Can you work these out from the model? Positions are in its coordinate system, mm. A direction names the side the tool comes from. Give positions to 0.01 mm unless a question says otherwise; leave off trailing zeros. Loops run counter-clockwise (first coordinate to the right, second up) from the corner with the lowest first, then second, coordinate; pieces in that order, holes last. Notation, with made-up numbers: (6.5, 57) -> (39.5, 57) arc R21 cw to (39.5, 94) -> close; hole circle Ø9 at (-36.75, 71.25). An arc over 180 degrees is marked (long way). Use CSV: the item, a comma, the result in double quotes.
from build123d import *

# Parameters (mm, degrees)
F1_DEPTH  = 35
F2_R      = 1
F4_DEPTH  = 25
F6_DEPTH  = 25
F8_DEPTH  = 25
F10_DEPTH = 25


with BuildPart() as f1:
    # F0 (on Top) → F1 (new body)
    with BuildSketch(Plane.XY):
        Polygon((1.5, 17.5), (1.5, 112.5), (-1.5, 112.5), (-1.5, 17.5), (-74, 17.5), (-74, 14.5), (-1.5, 14.5), (-1.5, -14.5), (-74, -14.5), (-74, -17.5), (-1.5, -17.5), (-1.5, -112.5), (1.5, -112.5), (1.5, -17.5), (74, -17.5), (74, -14.5), (1.5, -14.5), (1.5, 14.5), (74, 14.5), (74, 17.5), align=None)
    extrude(amount=F1_DEPTH)

    # F2
    f2_edges = [f1.edges().sort_by_distance(p)[0] for p in [
        (-37.75, 14.5, 35),
        (-1.5, 65, 35),
        (-37.75, 17.5, 35),
        (1.5, 65, 35),
        (37.75, 17.5, 35),
        (37.75, 14.5, 35),
        (1.5, 0, 35),
        (-1.5, 0, 35),
        (-37.75, -14.5, 35),
        (-37.75, -17.5, 35),
        (37.75, -14.5, 35),
        (37.75, -17.5, 35),
        (-1.5, -65, 35),
        (1.5, -65, 35),
    ]]
    fillet(f2_edges, radius=F2_R)

    # F3 (on face) → F4 (cut)
    with BuildSketch(Plane.XZ.offset(17.5)):
        with BuildLine():
            ThreePointArc((-46.6319660113, 34), (-37.75, 25.1180339887), (-28.8680339887, 34))
            Line((-28.8680339887, 34), (-46.6319660113, 34))
        make_face()
        with BuildLine():
            Line((-46.6319660113, 34), (-28.8680339887, 34))
            ThreePointArc((-28.8680339887, 34), (-37.75, 42.8819660113), (-46.6319660113, 34))
        make_face()
    extrude(amount=-F4_DEPTH, mode=Mode.SUBTRACT)

    # F5 (on face) → F6 (cut)
    with BuildSketch(Plane.XZ.offset(-14.5)):
        with BuildLine():
            ThreePointArc((-47.75, 34), (-37.75, 24), (-27.75, 34))
            Line((-27.75, 34), (-47.75, 34))
        make_face()
        with BuildLine():
            Line((-47.75, 34), (-27.75, 34))
            ThreePointArc((-27.75, 34), (-37.75, 44), (-47.75, 34))
        make_face()
    extrude(amount=-F6_DEPTH, mode=Mode.SUBTRACT)

    # F7 (on face) → F8 (cut)
    with BuildSketch(Plane.XZ.offset(17.5)):
        with BuildLine():
            Line((27.75, 34), (47.75, 34))
            ThreePointArc((47.75, 34), (37.75, 44), (27.75, 34))
        make_face()
        with BuildLine():
            ThreePointArc((27.75, 34), (37.75, 24), (47.75, 34))
            Line((47.75, 34), (27.75, 34))
        make_face()
    extrude(amount=-F8_DEPTH, mode=Mode.SUBTRACT)

    # F9 (on face) → F10 (cut)
    with BuildSketch(Plane.XZ.offset(-14.5)):
        with BuildLine():
            Line((27.75, 34), (47.75, 34))
            ThreePointArc((47.75, 34), (37.75, 44), (27.75, 34))
        make_face()
        with BuildLine():
            ThreePointArc((27.75, 34), (37.75, 24), (47.75, 34))
            Line((47.75, 34), (27.75, 34))
        make_face()
    extrude(amount=-F10_DEPTH, mode=Mode.SUBTRACT)


solid = f1.part
(1) If we section it at B-B, the plane z = 17: Write out the boundary of the cut face in (x, y), then the cut area to 4 significant figures.
Answer sheet:
outline,"(-74, -17.5) -> (-1.5, -17.5) -> (-1.5, -112.5) -> (1.5, -112.5) -> (1.5, -17.5) -> (74, -17.5) -> (74, -14.5) -> (1.5, -14.5) -> (1.5, 14.5) -> (74, 14.5) -> (74, 17.5) -> (1.5, 17.5) -> (1.5, 112.5) -> (-1.5, 112.5) -> (-1.5, 17.5) -> (-74, 17.5) -> (-74, 14.5) -> (-1.5, 14.5) -> (-1.5, -14.5) -> (-74, -14.5) -> close"
area,"1,545 mm2"
(2) Which directions (+Z, -Z, +X, -X, +Y, -Y) give clear straight access to the entire face, cutting with the end or side of a thin tool? Please do faces 1 (the face through (-37, 17.5, 17)), 2 (the face through (37, -17.5, 17)), 3 (the face through (-1.5, -64, 17)).
Answer sheet:
face 1,"+Z, -Z, -X, +Y"
face 2,"+Z, -Z, +X, -Y"
face 3,"+Z, -Z, -X, -Y"
(3) If we section it at A-A, the plane x = 37.75: Write out the boundary of the cut face in (y, z), then the cut area to 3 significant figures.
Answer sheet:
outline,"(-17.5, 0) -> (-14.5, 0) -> (-14.5, 24) -> (-17.5, 24) -> close; (14.5, 0) -> (17.5, 0) -> (17.5, 24) -> (14.5, 24) -> close"
area,"144 mm2"
(4) Will these pins go through, and if not, where does the flat tip stop? pin 1 Ø17 at (x, z) = (-27.5, 13) entering from -Y; pin 2 Ø10 at (y, z) = (-63, 11) entering from -X; pin 3 Ø17 at (y, z) = (-62.5, 19) entering from +X.
Answer sheet:
pin 1,"stops at y = -17.5"
pin 2,"stops at x = -1.5"
pin 3,"stops at x = 1.5"
(5) If we section it at C-C, the plane x = -58: Write out the boundary of the cut face in (y, z), then the cut area to 3 significant figures.
Answer sheet:
outline,"(-17.5, 0) -> (-14.5, 0) -> (-14.5, 34) arc R1 ccw to (-15.5, 35) -> (-16.5, 35) arc R1 ccw to (-17.5, 34) -> close; (14.5, 0) -> (17.5, 0) -> (17.5, 34) arc R1 ccw to (16.5, 35) -> (15.5, 35) arc R1 ccw to (14.5, 34) -> close"
area,"209 mm2"
(6) We'd pull the mould along Y, two halves only. Please class faces 4 (the face through (-38, -17.5, 17)), 5 (the face through (37.516, -16.021, 24.003)), 6 (the face through (-37, -14.5, 17)), 7 (the face through (38, 17.5, 17)): released by +Y, released by -Y, zero draft, split by the parting line, or undercut.
Answer sheet:
face 4,"released by -Y"
face 5,"zero draft"
face 6,"undercut"
face 7,"released by +Y"
(7) If I drill on L1, parallel to X at y = 16.9, z = 34; L2, parallel to X at y = -16.5, z = 34; L3, parallel to Y at x = 21, z = 9, over which ranges is the centre line in solid material (lowest first)? Write a range as from..to.
Answer sheet:
L1,"x = -74..-47.75, -27.75..27.75, 47.75..74"
L2,"x = -74..-46.63, -28.87..27.75, 47.75..74"
L3,"y = -17.5..-14.5, 14.5..17.5"
(8) If we section it at D-D, the plane y = -69.5: Write out the boundary of the cut face in (x, z).
Answer sheet:
outline,"(-1.5, 0) -> (1.5, 0) -> (1.5, 34) arc R1 ccw to (0.5, 35) -> (-0.5, 35) arc R1 ccw to (-1.5, 34) -> close"
